Can you work these out from the model? Positions are in its coordinate system, mm. A direction names the side the tool comes from. Round coordinates to 2 decimals unless told otherwise and drop trailing zeros. Write each loop counter-clockwise with the first axis right and the second up, starting at its lowest first coordinate (ties: lowest second). Pieces come first, ordered by that corner, then holes. Notation, with made-up numbers: M 68,9.25 L 82,9.25 A15 ccw 82,38.25 Z; hole C 61.5,-23 d6. An arc over 180 degrees is marked long. Answer as a JSON object with one key per item and string values. Group by question number.
1) Suppose I cut it at B-B, the plane z = 0. Write out the boundary of the cut face in (x, y).
2) On a 3-axis mill with a long thin cutter (end or side, diameter ignored), from which of +Z, -Z, +X, -X, +Y, -Y can I reach the whole of each face in a straight line? I mean faces 5 (the flat face through (0, 0, 0)), 6 (the cylindrical face through (-0.617, 0.188, -2.777)), 7 (the flat face through (1, 0, 1)). Say none if no direction works.
3) Suppose I cut it at C-C, the plane y = -2.75. Write out the boundary of the cut face in (x, z), and give its area (3 significant figures).
4) If we mould it in two halves opening along X, with no side actions, what happens to faces 1 (the flat face through (0, -8, 0)), 2 (the flat face through (0.502, 0.814, 0.854)), 3 (the flat face through (0.991, 1, 0)), 4 (the cylindrical face through (0.27, -3.94, -1.23))? For each: +X half, -X half, draft (parallel to the pull), parting line (faces both ways), or undercut.
5) Suppose I cut it at A-A, the plane y = 0.25. Write out the boundary of the cut face in (x, z).
6) Please list where these lines run through material, in increasing order: L1, parallel to Y at x = -0.8, z = 0.5; L2, parallel to Y at x = -1.3, z = -0.95; L3, parallel to Z at x = 0.7, y = 0.25. Write a range as [from, to].
7) I'm going to push flat-ended pins straight in: pin 1 Ø1.5 at (y, z) = (-2, 1.5) entering from -X; pin 2 Ø0.9 at (y, z) = (1, 0) entering from -X; pin 3 Ø3 at (x, y) = (-2, -2.5) entering from +Z. Where does each tip first touch, or does it pass through?
Autodesk Inventor part; units mm, degrees
ref_plane "YZ Plane" through (0, 0, 0) normal (1, 0, 0) x (0, 1, 0)
ref_plane "XZ Plane" through (0, 0, 0) normal (0, 1, 0) x (-1, 0, 0)
ref_plane "XY Plane" through (0, 0, 0) normal (0, 0, 1) x (1, 0, 0)
sketch "Sketch1" plane through (0, 0, 0) normal (0, 1, 0) x (-1, 0, 0)
  circle A0 centre (0, 0) radius 1.2573
  dimension "d0" = 2.5146
extrude "Extrusion1" add sketch "Sketch1" against normal blind 8
sketch "Sketch2" plane through (0, 0, 0) normal (0, 1, 0) x (1, 0, 0)
  circle A0 centre (0, 0) radius 1.2573
  circle A1 centre (0, 0) radius 2.8448
  line L0 (0, 0) -> (0.9906, 0)
  line L1 (0.9906, -0.5719) -> (0, -1.1438)
  line L2 (0, -1.1438) -> (-0.9906, -0.5719)
  line L3 (-0.9906, -0.5719) -> (-0.9906, 0.5719)
  line L4 (-0.9906, 0.5719) -> (0, 1.1438)
  line L5 (0, 1.1438) -> (0.9906, 0.5719)
  line L6 (0.9906, 0.5719) -> (0.9906, -0.5719)
  dimension "d7" = 0.9906
extrude "Extrusion2" add sketch "Sketch2" along normal blind 1.651 contours A0 | A1
fillet "Fillet1" radius 1.27 1 edges at (-2.8448, 1.651, 0)
thread "Thread1"
properties part number "m3x8"
Results:
{
 "1": {"outline": "M -2.84,0 L -1.26,0 L -1.26,-8 L 1.26,-8 L 1.26,0 L 2.84,0 L 2.84,0.38 A1.27 ccw 1.57,1.65 L 0.99,1.65 L 0.99,0 L -0.99,0 L -0.99,1.65 L -1.57,1.65 A1.27 ccw -2.84,0.38 Z"},
 "2": {"face 5": "+Y", "face 6": "+Y, -Y", "face 7": "-Y"},
 "3": {"outline": "C 0,0 d2.51", "area": "4.97 mm^2"},
 "4": {"face 1": "draft", "face 2": "undercut", "face 3": "undercut", "face 4": "parting line"},
 "5": {"outline": "C 0,0 d5.69; hole M -0.99,-0.57 L 0,-1.14 L 0.99,-0.57 L 0.99,0.57 L 0,1.14 L -0.99,0.57 Z"},
 "6": {"L1": "[-8, 0]", "L2": "[0, 1.65]", "L3": "[-2.76, -0.74], [0.74, 2.76]"},
 "7": {"pin 1": "x = -1.01", "pin 2": "x = -2.83", "pin 3": "z = 1.15"}
}
